Verification items for the finished model (mm, model axes). A direction names the side the tool comes from. Coordinates: 2 decimals unless noted, no trailing zeros. Order: outer loops, then holes, each group sorted by start corner. A loop starts at its lowest first (then second) coordinate and runs counter-clockwise, first axis right, second up. Notation, with made-up numbers: M 48,81 L 83,81 A25 cw 83,120 Z; hole C -18,-6 d6. An arc over 180 degrees is marked long. Return JSON: item names as keys, results as strings. Group by question number.
Q1. Thickness scan on probe 1 along Z at (x, y) = (-9.5, -43.5) (3 decimals); probe 2 along Z at (x, y) = (59, 2.5); probe 3 along X at (y, z) = (-10.5, 17.5) (3 decimals). Record the ranges inside material, lowest first.
Q2. Section check B-B, the plane x = 61.5. Enter the section's corners in (y, z).
Q3. Access from +Z, -Z, +X, -X, +Y, -Y to the whole of each face (thin tool, end or side, straight path). Record for faces 1 (the face through (91, 0, 38.1)), 2 (the face through (48, -25.4, 42)), 3 (the face through (48, 25.4, 42)).
Q4. Section check A-A, the plane y = -45. Enter the section's corners in (x, z) (3 decimals).
Q5. Go/stop test with flat-tipped pins: pin 1 Ø8 at (y, z) = (-13, 9.5) entering from +X (3 decimals); pin 2 Ø6 at (x, y) = (98.5, -29.5) entering from +Z; pin 3 Ø1.5 at (x, y) = (64.5, 16) entering from -Z; pin 4 Ø16 at (x, y) = (78, -10.5) entering from -Z. Record where each tip stops, or that it passes through.
from build123d import *

# Parameters (mm, degrees)
F1_DEPTH = 63.5
F0_W     = 24.486841
F0_H     = 19.05
F2_DEPTH = 25.4
F3_DEPTH = 7.9375
F5_R     = 6.35


with BuildPart() as f1:
    # F0 (on Front) → F1 (new body, symmetric)
    with BuildSketch(Plane.XZ):
        Polygon((22.225, 9.525), (-41.275, 9.525), (-41.275, -9.525), (41.275, -9.525), (41.275, 9.525), align=None)
    extrude(amount=F1_DEPTH, both=True)

    # F0 (on Front) → F2 (join, symmetric)
    with BuildSketch(Plane.XZ):
        with BuildLine():
            Line((22.225, 27.024607), (22.225, 9.525))
            Line((22.225, 9.525), (41.275, 9.525))
            Line((41.275, 9.525), (41.275, 27.024607))
            ThreePointArc((41.275, 27.024607), (46.240227, 38.556844), (58.029959, 42.8752))
            Line((58.029959, 42.8752), (65.447114, 42.8752))
            Line((65.447114, 42.8752), (65.447114, 61.9252))
            Line((65.447114, 61.9252), (58.455464, 61.9252))
            add(Edge.make_bspline(
                [(49.01163, 60.988154), (52.041988, 61.446427), (55.185381, 61.764423), (58.455464, 61.9252)],
                knots=[104.564463, 104.564463, 104.564463, 104.564463, 112.658539, 112.658539, 112.658539, 112.658539], degree=3))
            ThreePointArc((49.01163, 60.988154), (29.727489, 48.652402), (22.225, 27.024607))
        make_face()
        with Locations((77.690534, 52.4002)):
            Rectangle(F0_W, F0_H)
    extrude(amount=F2_DEPTH, both=True)

    # F0 (on Front) → F3 (join, symmetric)
    with BuildSketch(Plane.XZ):
        with BuildLine():
            add(Edge.make_bspline(
                [(-41.275, 9.525), (-10.419927, 25.736817), (9.863519, 55.0679), (49.01163, 60.988154)],
                knots=[0, 0, 0, 0, 104.564463, 104.564463, 104.564463, 104.564463], degree=3))
            Line((-41.275, 9.525), (22.225, 9.525))
            Line((22.225, 9.525), (22.225, 27.024607))
            ThreePointArc((22.225, 27.024607), (29.727489, 48.652402), (49.01163, 60.988154))
        make_face()
    extrude(amount=F3_DEPTH, both=True)

    # F0 (on Front) → F4 (revolve)
    with BuildSketch(Plane.XZ):
        Polygon((116.247114, 66.675), (90.847114, 66.675), (90.847114, 52.3875), (90.847114, 38.1), (116.247114, 38.1), align=None)
    revolve(axis=Axis((90.847114, 0, 52.3875), (0, 0, 1)))

    # F5
    f5_edges = [f1.edges().sort_by_distance(p)[0] for p in [
        (41.275, -63.5, 0),
        (-41.275, -63.5, 0),
        (41.275, 63.5, 0),
        (-41.275, 63.5, 0),
    ]]
    fillet(f5_edges, radius=F5_R)


solid = f1.part
Numbers:
{
 "1": {"probe 1": "z = -9.525 to 9.525", "probe 2": "z = 42.88 to 61.93", "probe 3": "x = 22.225 to 41.275"},
 "2": {"outline": "M -25.4,42.88 L 25.4,42.88 L 25.4,61.93 L -25.4,61.93 Z"},
 "3": {"face 1": "-Z, +X, +Y, -Y", "face 2": "+Z, +X, -X, -Y", "face 3": "+Z, +X, -X, +Y"},
 "4": {"outline": "M -41.275,-9.525 L 41.275,-9.525 L 41.275,9.525 L -41.275,9.525 Z"},
 "5": {"pin 1": "stops at x = 41.275", "pin 2": "passes through", "pin 3": "stops at z = 42.88", "pin 4": "stops at z = 38.1"}
}
